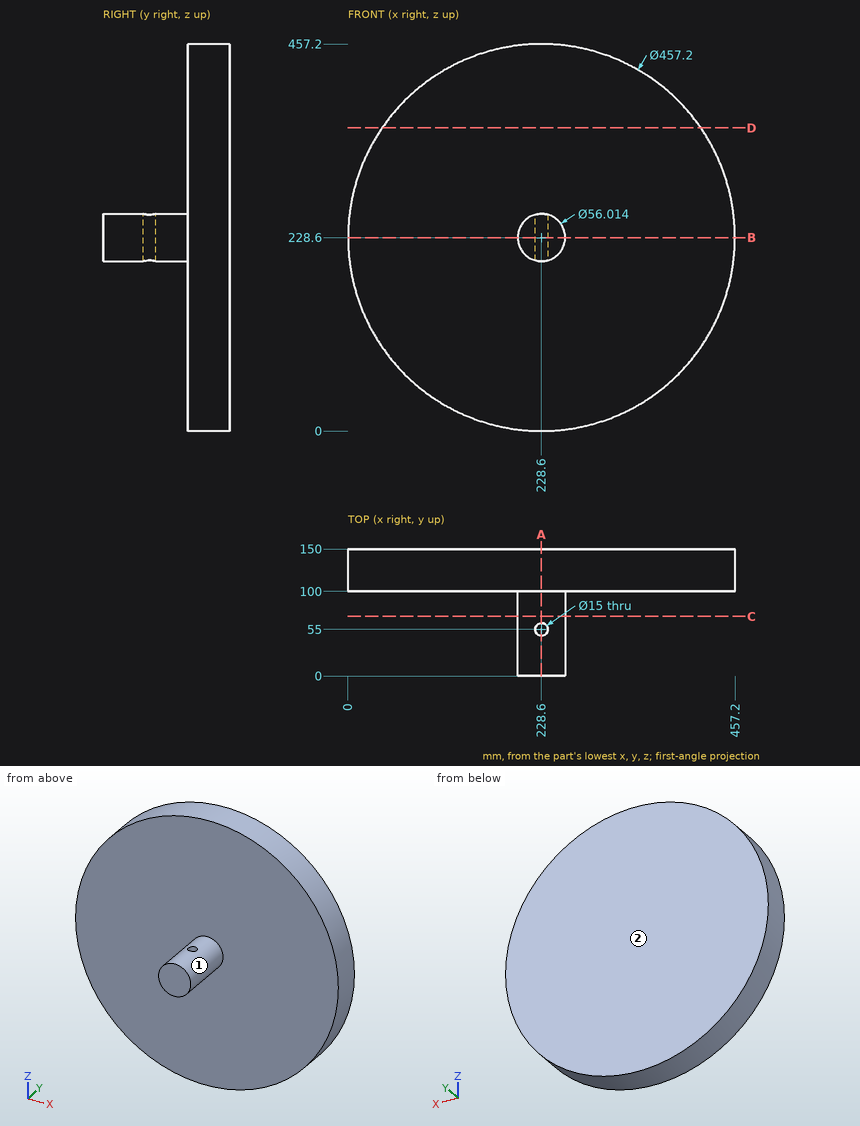
The figure shows three views and two pictorial views of one solid part (mm, origin at its lowest corner). Answer the questions. A direction names the side the tool comes from. Round coordinates to 2 decimals unless told otherwise and drop trailing zeros. Write each loop counter-clockwise with the first axis right and the second up, starting at its lowest first coordinate (ties: lowest second). Pieces come first, ordered by that corner, then holes. Notation, with made-up numbers: (65, -15) - (96, -15) arc R4 ccw to (96, -10) - close; hole circle Ø6 at (40, 24.5). An arc over 180 degrees is marked (long way). Answer in a Markdown table with one row per item. Add a question column.
1. A cutting plane is placed at D-D, the plane z = 358. Determine the outline of the cut face in (x, y), and give its area (3 significant figures).
2. A cutting plane is placed at C-C, the plane y = 70.5. Determine the outline of the cut face in (x, z).
3. A cutting plane is placed at A-A, the plane x = 228.6. Determine the outline of the cut face in (y, z).
4. Given pin 1 (4 mm diameter, centred on x = 89, z = 311, fed in from -Y); pin 2 (2 mm diameter, centred on y = 118.5, z = 137.5, fed in from -X) (3 decimals); pin 3 (3 mm diameter, centred on x = 73, y = 124, fed in from +Z), each flat-ended and moving along its own axis, determine where each tip first touches the part or whether it passes through.
5. Find the intervals of material crossed by line 1 along Y through (x, z) = (228.6, 234.5); line 2 along Y through (x, z) = (279.5, 335); line 3 along Z through (x, y) = (226.5, 33), in increasing order. Write a range as from..to.
6. For the marked faces 1 and 2, determine the directions among +Z, -Z, +X, -X, +Y, -Y from which every point of the face is accessible in a straight line to the end or side of a thin tool.
7. A cutting plane is placed at B-B, the plane z = 228.6. Determine the outline of the cut face in (x, y), and give its area (3 significant figures).
Worked out:
| question | item | result |
|---|---|---|
| 1 | outline | (40.15, 100) - (417.05, 100) - (417.05, 150) - (40.15, 150) - close |
| 1 | area | 18,800 mm^2 |
| 2 | outline | circle Ø56.01 at (228.6, 228.6) |
| 3 | outline | (0, 200.59) - (47.5, 200.59) - (47.5, 256.61) - (0, 256.61) - close; (62.5, 200.59) - (100, 200.59) - (100, 0) - (150, 0) - (150, 457.2) - (100, 457.2) - (100, 256.61) - (62.5, 256.61) - close |
| 4 | pin 1 | y = 100 |
| 4 | pin 2 | x = 18.505 |
| 4 | pin 3 | z = 397.45 |
| 5 | line 1 | 0..47.5, 62.5..150 |
| 5 | line 2 | 100..150 |
| 5 | line 3 | 200.67..256.53 |
| 6 | face 1 | -Y |
| 6 | face 2 | +Z, -Z, +X, -X, +Y |
| 7 | outline | (0, 100) - (200.59, 100) - (200.59, 0) - (256.61, 0) - (256.61, 100) - (457.2, 100) - (457.2, 150) - (0, 150) - close; hole circle Ø15 at (228.6, 55) |
| 7 | area | 28,300 mm^2 |
